Check sheet for the drawn part. Datum: minimum x, y, z corner. Units: mm. A direction names the side the tool comes from. Round coordinates to 2 decimals unless told otherwise and drop trailing zeros. Write each loop counter-clockwise with the first axis right and the second up, starting at its lowest first coordinate (ties: lowest second). Pieces come first, ordered by that corner, then holes. Notation, with made-up numbers: M 88.25,9 L 130.25,9 A8 ccw 130.25,13 Z; hole C 46.25,-1.75 d11. An arc over 180 degrees is marked long. Put each result on its own line as item: value.
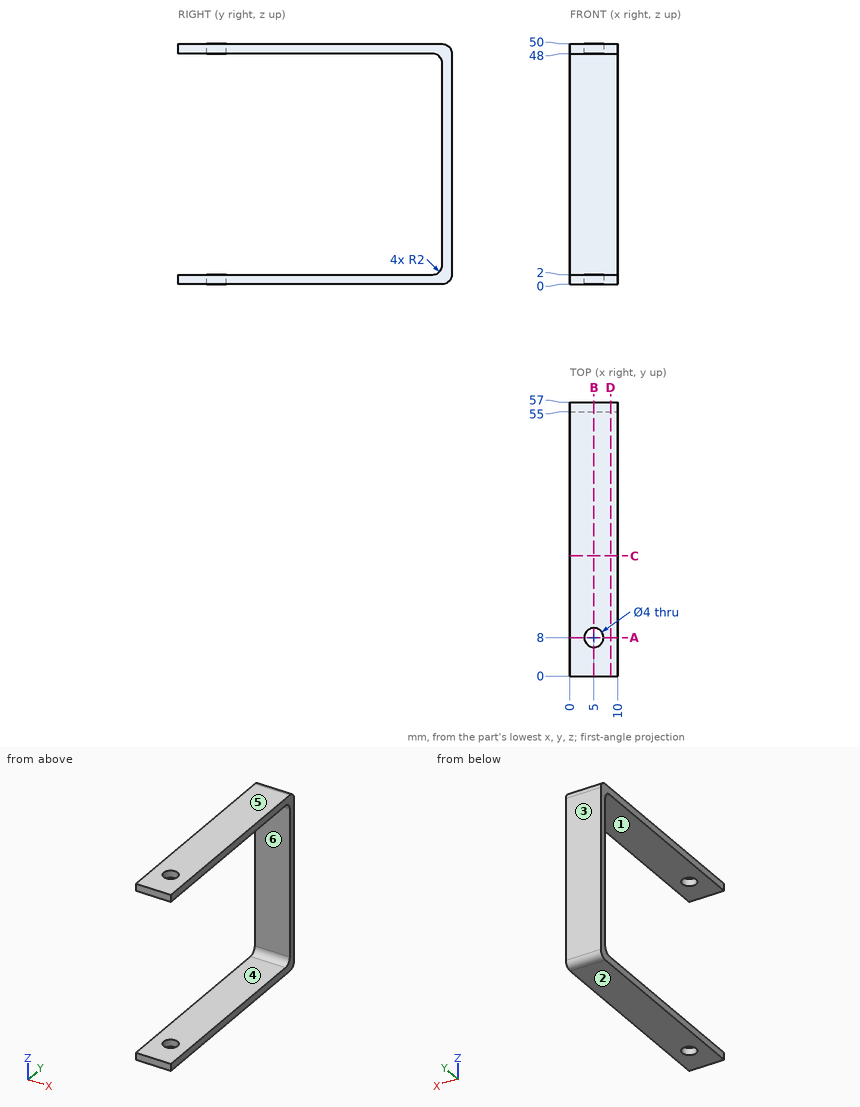
1. Cross-section at C-C (y = 25). Enter the section's corners in (x, z).
Computed values:
outline: M 0,0 L 10,0 L 10,2 L 0,2 Z; M 0,48 L 10,48 L 10,50 L 0,50 Z
2. Scan lines: probe 1 along Z at (x, y) = (7, 5); probe 2 along Y at (x, z) = (5, 49.5); probe 3 along Y at (x, z) = (2.75, 27). Record each from-to range of solid material in increasing order.
Computed values:
probe 1: z = 0 to 2, 48 to 50
probe 2: y = 0 to 6, 10 to 56.32
probe 3: y = 55 to 57
3. Depth check by flat-ended pin: pin 1 Ø5 at (x, z) = (5, 27) entering from -Y; pin 2 Ø3 at (x, y) = (5, 8) entering from -Z. Enter the tip coordinate at first touch or a pass-through.
Computed values:
pin 1: stops at y = 55
pin 2: passes through
4. Release check for a two-part mould opening along Z. For the marked faces 1, 2, 3 and 4 record: +Z half, -Z half, draft (parallel to the pull), parting line (faces both ways), or undercut.
Computed values:
face 1: undercut
face 2: -Z half
face 3: draft
face 4: undercut
5. Access from +Z, -Z, +X, -X, +Y, -Y to the whole of each face (thin tool, end or side, straight path). Record for the marked faces 5 and 6.
Computed values:
face 5: +Z, +X, -X, +Y, -Y
face 6: +X, -X, -Y
6. Cross-section at A-A (y = 8). Enter the section's corners in (x, z).
Computed values:
outline: M 0,0 L 3,0 L 3,2 L 0,2 Z; M 0,48 L 3,48 L 3,50 L 0,50 Z; M 7,0 L 10,0 L 10,2 L 7,2 Z; M 7,48 L 10,48 L 10,50 L 7,50 Z
7. Cross-section at B-B (x = 5). Enter the section's corners in (y, z), then the cut area to 3 significant figures.
Computed values:
outline: M 0,0 L 6,0 L 6,2 L 0,2 Z; M 0,48 L 6,48 L 6,50 L 0,50 Z; M 10,0 L 55,0 A2 ccw 57,2 L 57,48 A2 ccw 55,50 L 10,50 L 10,48 L 53,48 A2 cw 55,46 L 55,4 A2 cw 53,2 L 10,2 Z
area: 304 mm2
8. Cross-section at D-D (x = 8.5). Enter the section's corners in (y, z), then the cut area to 3 significant figures.
Computed values:
outline: M 0,0 L 55,0 A2 ccw 57,2 L 57,48 A2 ccw 55,50 L 0,50 L 0,48 L 53,48 A2 cw 55,46 L 55,4 A2 cw 53,2 L 0,2 Z
area: 320 mm2
